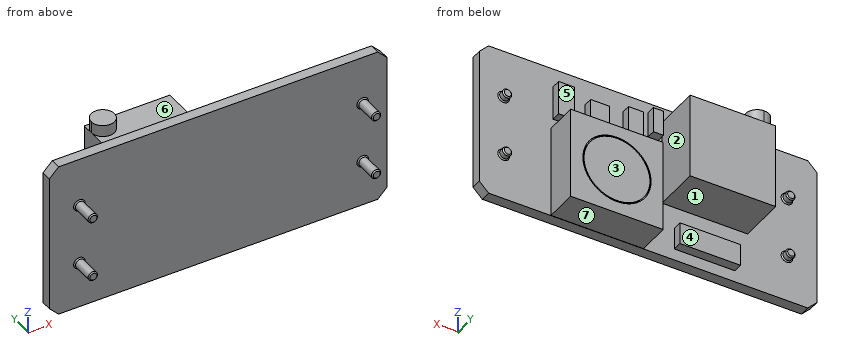
```python
from build123d import *

# Parameters (mm, degrees)
SKETCH1_W                = 37.084
SKETCH1_H                = 17.145
BOSS_EXTRUDE1_DEPTH      = 1.143
BOSS_EXTRUDE2_DEPTH      = 0.762
BOSS_EXTRUDE2_DEPTH_BACK = 3.683
SKETCH2_R                = 0.508
CHAMFER1_SIZE            = 0.127
SKETCH3_W                = 9.398
SKETCH3_H                = 9.398
BOSS_EXTRUDE3_DEPTH      = 5.08
BOSS_EXTRUDE4_DEPTH      = 3.556
BOSS_EXTRUDE5_DEPTH      = 1.27
SKETCH5_R                = 3.7465
SKETCH5_R_2              = 3.6195
CUT_EXTRUDE1_DEPTH       = 0.127
SKETCH6_W                = 6.657539154
SKETCH6_H                = 2.406121488
SKETCH6_W_2              = 1.664384789
SKETCH6_H_2              = 3.762956913
SKETCH6_W_3              = 1.736749344
SKETCH6_W_4              = 2.098572125
SKETCH6_H_3              = 2.460394905
SKETCH6_W_5              = 1.10355948
SKETCH6_H_4              = 2.804126546
BOSS_EXTRUDE6_DEPTH      = 1.016
CHAMFER2_SIZE            = 1.016
SKETCH7_W                = 10.16
SKETCH7_H                = 3.556
CUT_EXTRUDE2_DEPTH       = 0.0254


with BuildPart() as part:
    # Sketch1 → Boss-Extrude1 (new body)
    with BuildSketch(Plane(origin=(0, 0, 0), x_dir=(1, 0, 0), z_dir=(0, 1, 0))):
        with Locations((18.542, 8.5725)):
            Rectangle(SKETCH1_W, SKETCH1_H)
    extrude(amount=BOSS_EXTRUDE1_DEPTH)

    # Sketch2 → Boss-Extrude2 (add, two sides: drawn at the far end of the back side and taken through both)
    with BuildSketch(Plane(origin=(0, 1.143, 0), x_dir=(1, 0, 0), z_dir=(0, 1, 0)).offset(-BOSS_EXTRUDE2_DEPTH_BACK)):
        with Locations(Location((3.302, 12.065, 0), (0, 0, 90))):
            Circle(SKETCH2_R)
        with Locations(Location((3.302, 5.334, 0), (0, 0, 90))):
            Circle(SKETCH2_R)
        with Locations(Location((34.417, 12.065, 0), (0, 0, 90))):
            Circle(SKETCH2_R)
        with Locations(Location((34.417, 5.334, 0), (0, 0, 90))):
            Circle(SKETCH2_R)
    extrude(amount=BOSS_EXTRUDE2_DEPTH + BOSS_EXTRUDE2_DEPTH_BACK)

    # Chamfer1
    chamfer1_edges = [part.edges().sort_by_distance(p)[0] for p in [
        (3.302, 1.143, -11.557),
        (3.302, 0, -11.557),
        (3.302, -2.54, -11.557),
        (3.302, 1.905, -11.557),
        (3.302, 1.143, -4.826),
        (3.302, 0, -4.826),
        (3.302, -2.54, -4.826),
        (3.302, 1.905, -4.826),
        (34.417, 1.143, -11.557),
        (34.417, 0, -11.557),
        (34.417, -2.54, -11.557),
        (34.417, 1.905, -11.557),
        (34.417, 1.143, -4.826),
        (34.417, 0, -4.826),
        (34.417, -2.54, -4.826),
        (34.417, 1.905, -4.826),
    ]]
    chamfer(chamfer1_edges, length=CHAMFER1_SIZE)

    # Sketch3 → Boss-Extrude3 (add)
    with BuildSketch(Plane(origin=(0, 1.143, 0), x_dir=(1, 0, 0), z_dir=(0, 1, 0))):
        with Locations((12.319, 6.35)):
            Rectangle(SKETCH3_W, SKETCH3_H)
    extrude(amount=BOSS_EXTRUDE3_DEPTH)

    # Sketch3_3 → Boss-Extrude4 (add)
    with BuildSketch(Plane(origin=(0, 1.143, 0), x_dir=(1, 0, 0), z_dir=(0, 1, 0))):
        Polygon((19.05, 17.145), (19.05, 11.049), (19.05, 6.985), (29.21, 6.985), (29.21, 17.145), align=None)
    extrude(amount=BOSS_EXTRUDE4_DEPTH)

    # Sketch4 → Boss-Extrude5 (add)
    with BuildSketch(Plane.XY.offset(-1.651)):
        with BuildLine():
            ThreePointArc((10.16, 4.953), (9.788025612, 5.851025612), (8.89, 6.223))
            Line((8.89, 6.223), (8.89, 4.953))
            Line((8.89, 4.953), (7.62, 4.953))
            ThreePointArc((7.62, 4.953), (8.89, 3.683), (10.16, 4.953))
        make_face()
        with BuildLine():
            Line((8.89, 4.953), (8.89, 6.223))
            ThreePointArc((8.89, 6.223), (7.991974388, 5.851025612), (7.62, 4.953))
            Line((7.62, 4.953), (8.89, 4.953))
        make_face()
    extrude(amount=BOSS_EXTRUDE5_DEPTH)

    # Sketch5 → Cut-Extrude1 (cut)
    with BuildSketch(Plane(origin=(0, 4.699, 0), x_dir=(1, 0, 0), z_dir=(0, 1, 0))):
        with Locations(Location((24.13, 12.065, 0), (0, 0, 270))):
            Circle(SKETCH5_R)
        with Locations(Location((24.13, 12.065, 0), (0, 0, 270))):
            Circle(SKETCH5_R_2, mode=Mode.SUBTRACT)
    extrude(amount=-CUT_EXTRUDE1_DEPTH, mode=Mode.SUBTRACT)

    # Sketch6 → Boss-Extrude6 (add)
    with BuildSketch(Plane(origin=(0, 1.143, 0), x_dir=(1, 0, 0), z_dir=(0, 1, 0))):
        with Locations((12.34578489, 14.660168276)):
            Rectangle(SKETCH6_W, SKETCH6_H)
        with Locations((20.486797444, 3.959259553)):
            Rectangle(SKETCH6_W_2, SKETCH6_H_2)
        with Locations((28.121258104, 3.959259553)):
            Rectangle(SKETCH6_W_3, SKETCH6_H_2)
        with Locations((24.430665747, 4.067806388)):
            Rectangle(SKETCH6_W_4, SKETCH6_H_3)
        with Locations((18.035448108, 2.55719628)):
            Rectangle(SKETCH6_W_5, SKETCH6_H_4)
    extrude(amount=BOSS_EXTRUDE6_DEPTH)

    # Chamfer2
    chamfer2_edges = [part.edges().sort_by_distance(p)[0] for p in [
        (0, 0.5715, -17.145),
        (37.084, 0.5715, -17.145),
        (37.084, 0.5715, 0),
        (0, 0.5715, 0),
    ]]
    chamfer(chamfer2_edges, length=CHAMFER2_SIZE)

    # Sketch7 → Cut-Extrude2 (cut)
    with BuildSketch(Plane(origin=(0, 0, -17.145), x_dir=(-1, 0, 0), z_dir=(0, 0, -1))):
        with Locations((-24.13, 2.921)):
            Rectangle(SKETCH7_W, SKETCH7_H)
    extrude(amount=-CUT_EXTRUDE2_DEPTH, mode=Mode.SUBTRACT)


solid = part.part
```
Could you check a few things on this model? Use its own coordinates, in mm. Face numbers are marked on the shaded views. A direction names the side the tool comes from. Give positions to 0.01 mm unless a question says otherwise; leave off trailing zeros. Order: outer loops, then holes, each group sorted by start corner. A loop starts at its lowest first (then second) coordinate and runs counter-clockwise, first axis right, second up.
Q1. Suppose I cut it at C-C, the plane y = -1. Write out the boundary of the cut face in (x, z) (3 decimals), and give its area (3 significant figures).
Q2. Suppose I cut it at D-D, the plane x = 31. Write out the boundary of the cut face in (y, z) (3 decimals).
Q3. If I drill on line 1 along Y through (x, z) = (5, -8.25); line 2 along X through (y, z) = (5.25, -5.75); line 3 along X through (y, z) = (4, -13.25), over which ranges is the centre line in solid material (lowest first)?
Q4. Suppose I cut it at A-A, the plane y = 3.25. Write out the boundary of the cut face in (x, z) (3 decimals), and give its area (3 significant figures).
Q5. I'm going to push flat-ended pins straight in: P1, Ø2, axis at x = 25, z = -10.5, coming from the +Y side; P2, Ø0.8, axis at x = 9.5, y = 5.5, coming from the +Z side; P3, Ø4, axis at y = -0.5, z = -9.5, coming from the +X side; P4, Ø0.6, axis at x = 34.5, z = -12, coming from the +Y side (3 decimals). Where does each tip first touch, or does it pass through?
Q6. We'd pull the mould along X, two halves only. Please class the marked faces 1 and 2: +X half, -X half, draft (parallel to the pull), parting line (faces both ways), or undercut.
Q7. For the marked faces 3, 4, 5, 6 and 7, which set-ups out of +Z, -Z, +X, -X, +Y, -Y let a thin tool reach every point of the face, with its end or its side?
Solution:
1. outline: circle Ø1.016 at (3.302, -12.065); circle Ø1.016 at (3.302, -5.334); circle Ø1.016 at (34.417, -12.065); circle Ø1.016 at (34.417, -5.334)
1. area: 3.24 mm2
2. outline: (0, -17.145) - (1.143, -17.145) - (1.143, 0) - (0, 0) - close
3. line 1: y = 0 to 1.14
3. line 2: x = 7.62 to 17.02
3. line 3: x = 19.05 to 29.21
4. outline: (7.62, -11.049) - (17.018, -11.049) - (17.018, -1.651) - (7.62, -1.651) - close; (19.05, -17.12) - (29.21, -17.12) - (29.21, -6.985) - (19.05, -6.985) - close
4. area: 191 mm2
5. P1: stops at y = 4.7
5. P2: stops at z = -0.38
5. P3: stops at x = 37.08
5. P4: stops at y = 1.905
6. face 1: draft
6. face 2: undercut
7. face 3: +Z, -Z, +X, +Y
7. face 4: -Z, -X, +Y
7. face 5: +Z, +X, +Y
7. face 6: +Z
7. face 7: -Z, +X, -X, +Y
